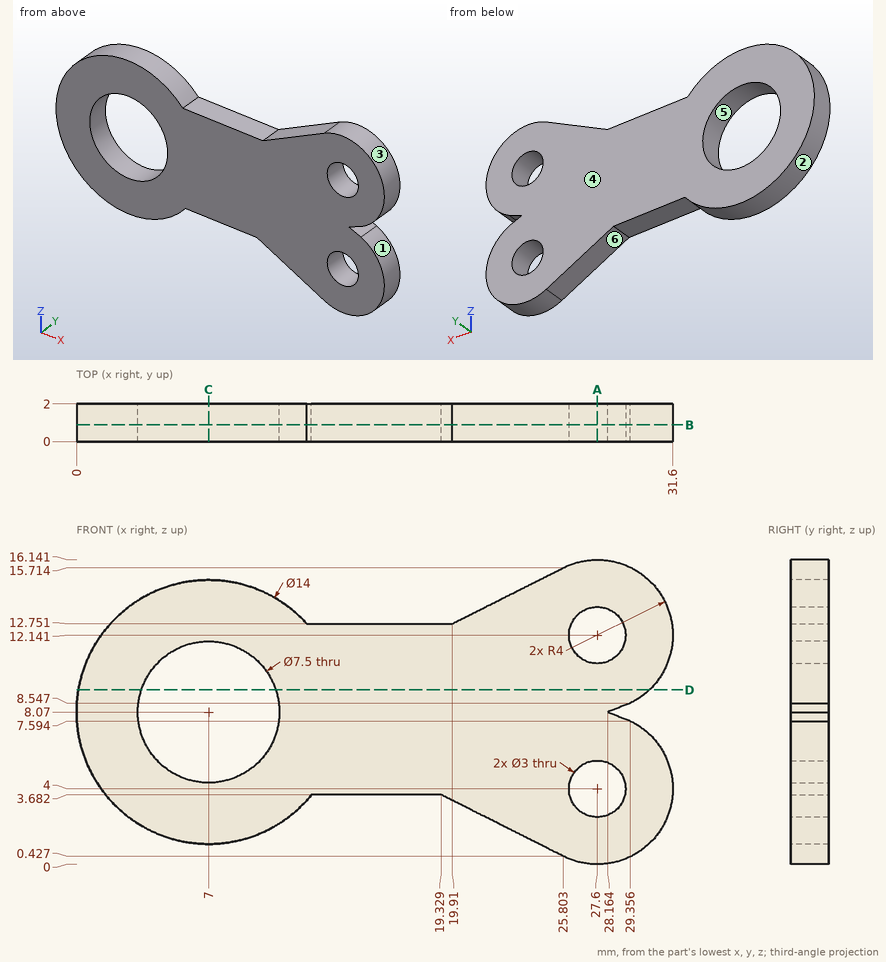
Drawing for the job (mm, zero at the part's lowest x, y, z). A direction names the side the tool comes from. Round coordinates to 2 decimals unless told otherwise and drop trailing zeros. Loops run counter-clockwise (first coordinate to the right, second up) from the corner with the lowest first, then second, coordinate; pieces in that order, holes last. Notation, with made-up numbers: (-39, -3.75) -> (5, -3.75) arc R28 cw to (5, 33.25) -> close; hole circle Ø4 at (87, 57.5). An arc over 180 degrees is marked (long way). Use one line per item in the form item = value. Start each with the question number.
Item 1: Two-plate mould, pull along Z, no slides. Class the marked faces 1, 2, 3 and 4: released by +Z, released by -Z, zero draft, split by the parting line, or undercut.
Item 2: Band-saw the part on B-B (y = 0.9). Give the number of separate pieces and of enclosed holes in the cut face, plus the area to 3 significant figures.
Item 3: Band-saw the part on A-A (x = 27.6). List the corners of the cut face in (y, z), plus the area to 3 significant figures.
Item 4: Band-saw the part on D-D (z = 9.25). List the corners of the cut face in (x, y) (1 decimal).
Item 5: Drop flat-ended pins along their axis: pin 1 Ø1 at (x, y) = (13.5, 0.5) entering from +Z; pin 2 Ø0.6 at (x, y) = (16.5, 0.5) entering from -Z. Give the stop position or say it passes through.
Item 6: Band-saw the part on C-C (x = 7). List the corners of the cut face in (y, z).
Item 7: Drill centre lines: line 1 along X through (y, z) = (1.85, 13.25) (1 decimal); line 2 along X through (y, z) = (1.25, 5.25) (1 decimal); line 3 along X through (y, z) = (0.75, 7.5) (1 decimal). Where is each one in solid material? Low to high.
Item 8: Tool access for the marked faces 5 and 6: list every direction of +Z, -Z, +X, -X, +Y, -Y with a clear straight run to the whole face (end or side of a thin tool).
Data:
q1.face_1 = undercut
q1.face_2 = split by the parting line
q1.face_3 = undercut
q1.face_4 = zero draft
q2.separate_pieces = 1
q2.enclosed_holes = 3
q2.area = 306 mm^2
q3.outline = (0, 0) -> (2, 0) -> (2, 2.5) -> (0, 2.5) -> close; (0, 5.5) -> (2, 5.5) -> (2, 10.64) -> (0, 10.64) -> close; (0, 13.64) -> (2, 13.64) -> (2, 16.14) -> (0, 16.14) -> close
q3.area = 20.3 mm^2
q4.outline = (0.1, 0) -> (3.4, 0) -> (3.4, 2) -> (0.1, 2) -> close; (10.6, 0) -> (30.4, 0) -> (30.4, 2) -> (10.6, 2) -> close
q5.pin_1 = 12.75
q5.pin_2 = 3.68
q6.outline = (0, 1.07) -> (2, 1.07) -> (2, 4.32) -> (0, 4.32) -> close; (0, 11.82) -> (2, 11.82) -> (2, 15.07) -> (0, 15.07) -> close
q7.line_1 = 2.3 to 11.7, 20.9 to 26.6, 28.6 to 31.4
q7.line_2 = 0.6 to 4.5, 9.5 to 26.8, 28.4 to 31.4
q7.line_3 = 0 to 3.3, 10.7 to 29.5
q8.face_5 = +Y, -Y
q8.face_6 = -Z, +Y, -Y
